For this review, take the finished solid that the model builds, in its own axes (mm). Face numbers are marked on the shaded views. A direction names the side the tool comes from. Coordinates: 2 decimals unless noted, no trailing zeros. Write each loop counter-clockwise with the first axis right and the second up, starting at its lowest first coordinate (ties: lowest second). Pieces come first, ordered by that corner, then holes. Notation, with made-up numbers: (18.25, 4) - (35.25, 4) arc R13 cw to (35.25, 27) - close; hole circle Ø5 at (-20, -38). An arc over 180 degrees is marked (long way). Use one line per item in the form item = value. Start each with the question number.
1) We need section D-D (y = 4.25). Give the boundary of the cut face in (x, z), plus the area to 3 significant figures.
2) Insertion check: P1, Ø1.3, axis at x = -3.1, z = -10.03, coming from the -Y side; P2, Ø1.5, axis at x = -1, y = 10, coming from the +Z side; P3, Ø2.5, axis at x = 0.5, z = 10.5, coming from the +Y side. Each pin has a flat end and moves straight along its axis. Give the tip position at first contact, or say it passes through.
3) We need section A-A (z = 0). Give the boundary of the cut face in (x, y), plus the area to 3 significant figures.
4) We need section C-C (y = 9.5). Give the boundary of the cut face in (x, z), plus the area to 3 significant figures.
5) Tool access review of the marked faces 4, 5, 6 and 7: name each direction out of +Z, -Z, +X, -X, +Y, -Y from which nothing blocks a thin tool from reaching the whole face with its end or side.
6) Mouldability with a two-part tool opening along X and no side actions: class the marked faces 1, 2 and 3 as pulls with the +X half, pulls with the -X half, needs draft (parallel to the pull), parting line crosses it, or undercut.
7) For L1, parallel to X at y = 13.3, z = 0; L2, parallel to X at y = 6.25, z = 0; L3, parallel to Z at x = -2.75, y = 4, list the stretches that pass through material, from the lowest coordinate up. Write a range as from..to.
8) We need section B-B (x = 0). Give the boundary of the cut face in (y, z), plus the area to 3 significant figures.
```python
from build123d import *

# Parameters (mm, degrees)
ENL_V_START                                   = -11.9
ENL_V_MAT_EXTRU_1_DEPTH                       = 11.9
ENL_V_START_2                                 = -5
ENL_V_MAT_EXTRU_2_DEPTH                       = 5
TROU_POUR_TARAUDAGE_POUR_TROU_TARAUD_M2_D     = 1.6
TROU_POUR_TARAUDAGE_POUR_TROU_TARAUD_M2_DEPTH = 8
TROU_POUR_TARAUDAGE_POUR_TROU_TARAUD_M2_TIP   = 0.480688495


with BuildPart() as part:
    # Esquisse1 → Révolution1 (revolve)
    with BuildSketch(Plane.XY, mode=Mode.PRIVATE) as r_volution1_sk:
        with BuildLine():
            Line((-8.4, 0), (-8.4, 11.4))
            ThreePointArc((-8.4, 11.4), (-8.107106781, 12.107106781), (-7.4, 12.4))
            Line((-7.4, 12.4), (-2.65, 12.4))
            Line((-2.65, 12.4), (-2.65, 13.9))
            Line((-2.65, 13.9), (-10.9, 13.9))
            ThreePointArc((-10.9, 13.9), (-11.960660172, 13.460660172), (-12.4, 12.4))
            Line((-12.4, 12.4), (-12.4, 0))
            Line((-12.4, 0), (-8.4, 0))
        make_face()
    revolve(r_volution1_sk.sketch.rotate(Axis((0, -3.661760917, 0), (0, 1, 0)), 270), axis=Axis((0, -3.661760917, 0), (0, 1, 0)))

    # Esquisse2 → Enlèv. mat.-Extru.1 (cut)
    with BuildSketch(Plane(origin=(0, 13.9, 0), x_dir=(1, 0, 0), z_dir=(0, 1, 0)).offset(ENL_V_START)):
        with BuildLine():
            Line((-10, 7.332121112), (-10, -7.332121112))
            ThreePointArc((-10, -7.332121112), (-12.4, 0), (-10, 7.332121112))
        make_face()
        with BuildLine():
            Line((10, 7.332121112), (10, -7.332121112))
            ThreePointArc((10, -7.332121112), (12.4, 0), (10, 7.332121112))
        make_face()
    extrude(amount=ENL_V_MAT_EXTRU_1_DEPTH, mode=Mode.SUBTRACT)

    # Esquisse3 → Enlèv. mat.-Extru.2 (cut)
    with BuildSketch(Plane(origin=(0, 13.9, 0), x_dir=(1, 0, 0), z_dir=(0, 1, 0)).offset(ENL_V_START_2)):
        with BuildLine():
            Line((-2.5, 9), (2.5, 9))
            Line((2.5, 9), (2.5, 12.145369488))
            ThreePointArc((2.5, 12.145369488), (0, 12.4), (-2.5, 12.145369488))
            Line((-2.5, 12.145369488), (-2.5, 9))
        make_face()
        with BuildLine():
            Line((2.5, -12.145369488), (2.5, -9))
            Line((2.5, -9), (-2.5, -9))
            Line((-2.5, -9), (-2.5, -12.145369488))
            ThreePointArc((-2.5, -12.145369488), (0, -12.4), (2.5, -12.145369488))
        make_face()
    extrude(amount=ENL_V_MAT_EXTRU_2_DEPTH, mode=Mode.SUBTRACT)

    # Trou pour taraudage pour trou taraudé M21
    with Locations(Plane(origin=(0, 0, 0), x_dir=(-1, 0, 0), z_dir=(0, -1, 0))):
        with Locations((-3.101869381, -10.034485853), (9.030088198, -5.363767998), (3.101869381, 10.034485853), (-9.030088198, 5.363767998)):
            Hole(TROU_POUR_TARAUDAGE_POUR_TROU_TARAUD_M2_D / 2, depth=TROU_POUR_TARAUDAGE_POUR_TROU_TARAUD_M2_DEPTH)
            with Locations((0, 0, -(TROU_POUR_TARAUDAGE_POUR_TROU_TARAUD_M2_DEPTH + TROU_POUR_TARAUDAGE_POUR_TROU_TARAUD_M2_TIP / 2))):  # 118° drill point
                Cone(0, TROU_POUR_TARAUDAGE_POUR_TROU_TARAUD_M2_D / 2, TROU_POUR_TARAUDAGE_POUR_TROU_TARAUD_M2_TIP, mode=Mode.SUBTRACT)


solid = part.part
```
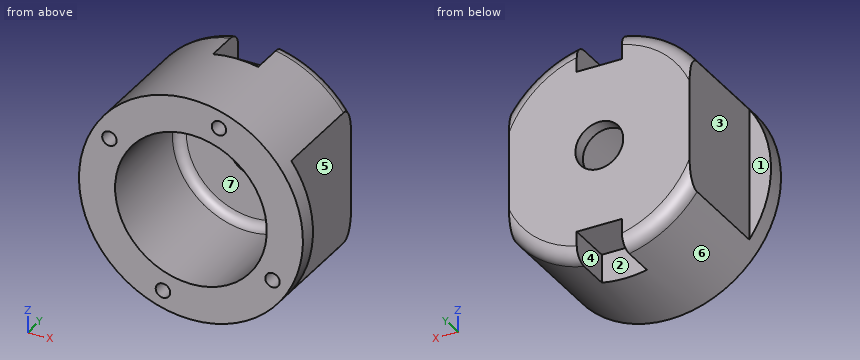
Determined:
q1.outline = (-10, -7.33) arc R12.4 ccw to (10, -7.33) - (10, 7.33) arc R12.4 ccw to (-10, 7.33) - close; hole circle Ø1.6 at (-9.03, 5.36); hole circle Ø16.8 at (0, 0); hole circle Ø1.6 at (-3.1, -10.03); hole circle Ø1.6 at (3.1, 10.03); hole circle Ø1.6 at (9.03, -5.36)
q1.area = 205 mm²
q2.P1 = 8.09
q2.P2 = 9
q2.P3 = 8.9
q3.outline = (-12.4, 0) - (-8.4, 0) - (-8.4, 11.4) arc R1 cw to (-7.4, 12.4) - (-2.65, 12.4) - (-2.65, 13.9) - (-10, 13.9) - (-10, 2) - (-12.4, 2) - close; (2.65, 12.4) - (7.4, 12.4) arc R1 cw to (8.4, 11.4) - (8.4, 0) - (12.4, 0) - (12.4, 2) - (10, 2) - (10, 13.9) - (2.65, 13.9) - close
q3.area = 71.8 mm²
q4.outline = (-10, -7.33) arc R12.4 ccw to (-2.5, -12.15) - (-2.5, -9) - (2.5, -9) - (2.5, -12.15) arc R12.4 ccw to (10, -7.33) - (10, 7.33) arc R12.4 ccw to (2.5, 12.15) - (2.5, 9) - (-2.5, 9) - (-2.5, 12.15) arc R12.4 ccw to (-10, 7.33) - close; hole circle Ø16.8 at (0, 0)
q4.area = 180 mm²
q5.face_4 = -Z, +Y
q5.face_5 = +Z, -Z, +X, +Y
q5.face_6 = +Y, -Y
q5.face_7 = -Y
q6.face_1 = needs draft
q6.face_2 = undercut
q6.face_3 = pulls with the -X half
q7.L1 = -10..-2.65, 2.65..10
q7.L2 = -10..-8.4, 8.4..10
q7.L3 = -12.09..-10.75, -9.32..-7.94, 7.94..12.09
q8.outline = (0, -12.4) - (8.9, -12.4) - (8.9, -9) - (13.9, -9) - (13.9, -2.65) - (12.4, -2.65) - (12.4, -7.4) arc R1 cw to (11.4, -8.4) - (0, -8.4) - close; (0, 8.4) - (11.4, 8.4) arc R1 cw to (12.4, 7.4) - (12.4, 2.65) - (13.9, 2.65) - (13.9, 9) - (8.9, 9) - (8.9, 12.4) - (0, 12.4) - close
q8.area = 94.9 mm²
